```python
from build123d import *

# Parameters (mm, degrees)
F0_R     = 40
F1_DEPTH = 100
F2_R     = 40
F3_DEPTH = 100
F4_R     = 40
F5_DEPTH = 100


with BuildPart() as f1:
    # F0 (on Front) → F1 (new body, symmetric)
    with BuildSketch(Plane.XZ):
        Circle(F0_R)
    extrude(amount=F1_DEPTH, both=True)

    # F2 (on Top) → F3 (intersect, symmetric)
    with BuildSketch(Plane.XY):
        Circle(F2_R)
    extrude(amount=F3_DEPTH, both=True, mode=Mode.INTERSECT)

    # F4 (on Right) → F5 (intersect, symmetric)
    with BuildSketch(Plane.YZ):
        Circle(F4_R)
    extrude(amount=F5_DEPTH, both=True, mode=Mode.INTERSECT)


solid = f1.part
```
Source: CAD feature listing. Evaluate the final solid. Frame: model axes, mm. Coordinates: 2 decimals unless noted, no trailing zeros. Loops run counter-clockwise (first coordinate to the right, second up) from the corner with the lowest first, then second, coordinate; pieces in that order, holes last. Notation, with made-up numbers: (38.5, 39.5) -> (97.5, 39.5) arc R18 cw to (97.5, 58.5) -> close; hole circle Ø4 at (46.5, -14.5). An arc over 180 degrees is marked (long way). One line per item, written item: value. Start each with the question number.
Q1. Section query C-C, the plane z = -31.5. Return the cut outline in (x, y), and give its area (3 significant figures).
Q2. Section query B-B, the plane y = 22. Return the cut outline in (x, z), and give its area (3 significant figures).
Q3. Section query D-D, the plane x = -30.5. Return the cut outline in (y, z).
Q4. Section query A-A, the plane x = 24. Return the cut outline in (y, z), and give its area (3 significant figures).
Q5. Line query: line 1 along X through (y, z) = (-21.5, -20); line 2 along X through (y, z) = (3.5, -14.5); line 3 along Z through (x, y) = (32.5, -15.5). Output: solid intervals per line, ascending.
Q6. Contact query for flat-ended pins moving along their axis: P1, Ø12, axis at y = -1.5, z = -30, coming from the -X side; P2, Ø3, axis at x = -16, z = 14, coming from the -Y side; P3, Ø10, axis at y = -23, z = 7, coming from the -X side. Output: stop coordinate, or through.
Results:
1. outline: (-24.65, -24.65) -> (24.65, -24.65) -> (24.65, 24.65) -> (-24.65, 24.65) -> close
1. area: 2,430 mm^2
2. outline: (-33.41, -22) arc R40 ccw to (-22, -33.41) -> (22, -33.41) arc R40 ccw to (33.41, -22) -> (33.41, 22) arc R40 ccw to (22, 33.41) -> (-22, 33.41) arc R40 ccw to (-33.41, 22) -> close
2. area: 4,240 mm^2
3. outline: (-25.88, -25.88) -> (25.88, -25.88) -> (25.88, 25.88) -> (-25.88, 25.88) -> close
4. outline: (-32, -24) arc R40 ccw to (-24, -32) -> (24, -32) arc R40 ccw to (32, -24) -> (32, 24) arc R40 ccw to (24, 32) -> (-24, 32) arc R40 ccw to (-32, 24) -> close
4. area: 3,980 mm^2
5. line 1: -33.73 to 33.73
5. line 2: -37.28 to 37.28
5. line 3: -23.32 to 23.32
6. P1: x = -32
6. P2: y = -37.28
6. P3: x = -35.72
